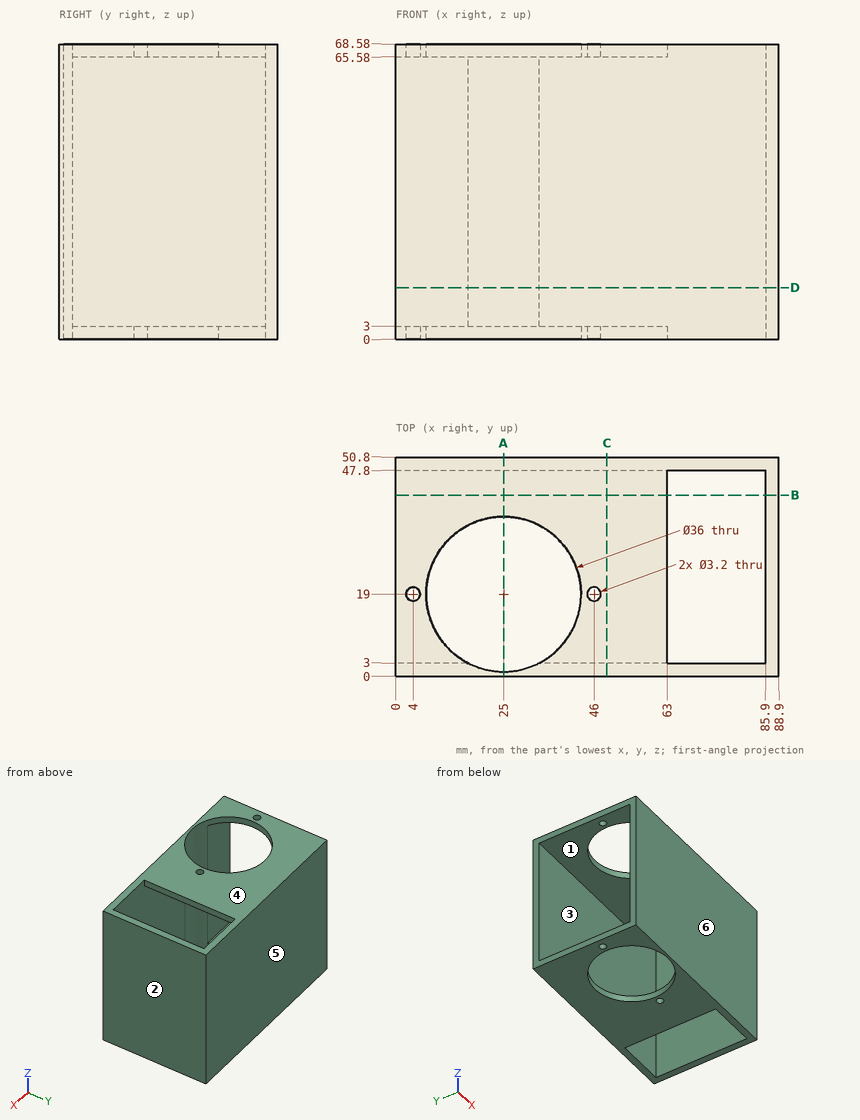
The drawing under review shows one solid part. Ordinate dimensions are in mm from its lowest x, y, z. A direction names the side the tool comes from. Round coordinates to 2 decimals unless told otherwise and drop trailing zeros. Write each loop counter-clockwise with the first axis right and the second up, starting at its lowest first coordinate (ties: lowest second). Pieces come first, ordered by that corner, then holes. Notation, with made-up numbers: (54.5, 44) -> (90.5, 44) arc R18 cw to (90.5, 76) -> close; hole circle Ø6 at (-20, 28). An arc over 180 degrees is marked (long way). One line per question, with ' | ' between items.
(1) Draft analysis for pull direction Y (two halves, no side actions). For the marked faces 3, 4, 5 and 6, state which applies: released by +Y, released by -Y, zero draft, split by the parting line, or undercut.
Result sheet:
face 3: undercut | face 4: zero draft | face 5: released by +Y | face 6: released by -Y
(2) Wall thickness on line 1 (X direction, y = 19, z = 0.95); line 2 (Z direction, x = 32.5, y = 40.5); line 3 (Y direction, x = 51.5, z = 41.5): over which ranges is each line inside the solid? List them lowest first. Write a range as [from, to].
Result sheet:
line 1: [0, 2.4], [5.6, 7], [43, 44.4], [47.6, 63], [85.9, 88.9] | line 2: [0, 3], [65.58, 68.58] | line 3: [0, 3], [47.8, 50.8]
(3) Take a section at A-A, the plane x = 25. State the section outline as (y, z) points, and give its area (3 significant figures).
Result sheet:
outline: (0, 0) -> (1, 0) -> (1, 68.58) -> (0, 68.58) -> close; (37, 0) -> (50.8, 0) -> (50.8, 68.58) -> (37, 68.58) -> (37, 65.58) -> (47.8, 65.58) -> (47.8, 3) -> (37, 3) -> close | area: 339 mm2
(4) Insertion check: P1, Ø13.5, axis at y = 34.5, z = 33.5, coming from the -X side. The pin has a flat end and moves straight along its axis. Give the tip position at first contact, or say it passes through.
Result sheet:
P1: x = 85.9
(5) Machinability: for the marked faces 1 and 2, which of the approach directions +Z, -Z, +X, -X, +Y, -Y give a long, thin tool a straight path to every point of the face, cutting with its end or side? Answer none if there is none.
Result sheet:
face 1: -X | face 2: +Z, -Z, +X, +Y, -Y
(6) Take a section at C-C, the plane x = 49. State the section outline as (y, z) points, and give its area (3 significant figures).
Result sheet:
outline: (0, 0) -> (50.8, 0) -> (50.8, 68.58) -> (0, 68.58) -> close; hole (3, 3) -> (47.8, 3) -> (47.8, 65.58) -> (3, 65.58) -> close | area: 680 mm2
(7) Take a section at B-B, the plane y = 42. State the section outline as (x, z) points.
Result sheet:
outline: (0, 0) -> (63, 0) -> (63, 3) -> (0, 3) -> close; (0, 65.58) -> (63, 65.58) -> (63, 68.58) -> (0, 68.58) -> close; (85.9, 0) -> (88.9, 0) -> (88.9, 68.58) -> (85.9, 68.58) -> close
(8) Take a section at D-D, the plane z = 12. State the section outline as (x, y) points, and give its area (3 significant figures).
Result sheet:
outline: (0, 0) -> (88.9, 0) -> (88.9, 50.8) -> (0, 50.8) -> (0, 47.8) -> (85.9, 47.8) -> (85.9, 3) -> (33.25, 3) arc R18 cw to (16.75, 3) -> (0, 3) -> close | area: 646 mm2
